Could you check a few things on this model? Use its own coordinates, in mm. A direction names the side the tool comes from. Give positions to 0.01 mm unless a question says otherwise; leave off trailing zeros. Order: outer loops, then holes, each group sorted by start corner. A loop starts at its lowest first (then second) coordinate and runs counter-clockwise, first axis right, second up. Notation, with made-up numbers: (19, 31) -> (66, 31) arc R23 cw to (66, 61) -> close; hole circle Ø9 at (-24, -18). An arc over 180 degrees is marked (long way). Write each question's results on one line, items separated by ' | '.
```python
from build123d import *

# Parameters (mm, degrees)
F0_R     = 17.5
F1_DEPTH = 5.5
F2_R     = 7.5
F3_DEPTH = 25
F4_R     = 15.2
F4_R_2   = 10.75
F5_DEPTH = 0.5


with BuildPart() as f1:
    # F0 (on Top) → F1 (new body)
    with BuildSketch(Plane.XY):
        Circle(F0_R)
    extrude(amount=F1_DEPTH)

    # F2 (on face) → F3 (cut)
    with BuildSketch(Plane.XY.offset(5.5)):
        Circle(F2_R)
    extrude(amount=-F3_DEPTH, mode=Mode.SUBTRACT)

    # F4 (on face) → F5 (cut)
    with BuildSketch(Plane.XY.offset(5.5)):
        Circle(F4_R)
        Circle(F4_R_2, mode=Mode.SUBTRACT)
    extrude(amount=-F5_DEPTH, mode=Mode.SUBTRACT)

    # F6: F1 across plane


with BuildPart() as f1_1:
    add(f1.part)
    add(f1.part.mirror(Plane.XY))


solid = f1_1.part
```
Q1. Suppose I cut it at A-A on y = 0. Please give me the cut outline in (x, z), and give its area (3 significant figures).
Here are the results:
outline: (-17.5, -5.5) -> (-15.2, -5.5) -> (-15.2, -5) -> (-10.75, -5) -> (-10.75, -5.5) -> (-7.5, -5.5) -> (-7.5, 5.5) -> (-10.75, 5.5) -> (-10.75, 5) -> (-15.2, 5) -> (-15.2, 5.5) -> (-17.5, 5.5) -> close; (7.5, -5.5) -> (10.75, -5.5) -> (10.75, -5) -> (15.2, -5) -> (15.2, -5.5) -> (17.5, -5.5) -> (17.5, 5.5) -> (15.2, 5.5) -> (15.2, 5) -> (10.75, 5) -> (10.75, 5.5) -> (7.5, 5.5) -> close | area: 211 mm²
Q2. Suppose I cut it at C-C on z = -1.75. Please give me the cut outline in (x, y), and give its area (3 significant figures).
Here are the results:
outline: circle Ø35 at (0, 0); hole circle Ø15 at (0, 0) | area: 785 mm²
Q3. For faces 4 (the flat face through (-3.6, 10.3, -5)), 5 (the flat face through (-3.6, 10.3, 5)), 6 (the flat face through (0, 16, 5.5)), which set-ups out of +Z, -Z, +X, -X, +Y, -Y let a thin tool reach every point of the face, with its end or its side?
Here are the results:
face 4: -Z | face 5: +Z | face 6: +Z, +X, -X, +Y, -Y
Q4. Thinking about a two-plate mould opening in X: for faces 1 (the flat face through (0, 16, -5.5)), 2 (the cylindrical face through (-13.887, -10.648, 0.077)), 3 (the cylindrical face through (-15.185, 0.668, 5.254)), which applies, +X half, -X half, draft (parallel to the pull), parting line (faces both ways), or undercut?
Here are the results:
face 1: draft | face 2: parting line | face 3: undercut
Q5. I'm going to push flat-ended pins straight in: pin 1 Ø3 at (y, z) = (8, -2.5) entering from +X; pin 2 Ø3 at (y, z) = (-3, 2) entering from +X; pin 3 Ø1.5 at (y, z) = (-13.5, 3.5) entering from +X. Where does each tip first touch, or does it pass through?
Here are the results:
pin 1: stops at x = 16.25 | pin 2: stops at x = 17.44 | pin 3: stops at x = 11.99
Q6. I need wall thicknesses on line 1 along Y through (x, z) = (0, -5.1); line 2 along Y through (x, z) = (0, -0.75); line 3 along X through (y, z) = (4, 5.25). Which ranges of each line are inside material? Lowest first, please.
Here are the results:
line 1: y = -17.5 to -15.2, -10.75 to -7.5, 7.5 to 10.75, 15.2 to 17.5 | line 2: y = -17.5 to -7.5, 7.5 to 17.5 | line 3: x = -17.04 to -14.66, -9.98 to -6.34, 6.34 to 9.98, 14.66 to 17.04
